```python
from build123d import *

# Parameters (mm, degrees)
F1_DEPTH = 4.75
F2_R     = 1.7
F3_DEPTH = 2.111
F4_R     = 1.6
F5_DEPTH = 2.111


with BuildPart() as f1:
    # F0 (on Front) → F1 (new body, symmetric)
    with BuildSketch(Plane.XZ):
        Polygon((-1.45, -4.75), (1.45, -4.75), (1.45, -3.15), (0.66, -3.15), (0.66, 0.05), (1.45, 0.05), (1.45, 1.65), (0.66, 1.65), (0.66, 4.75), (-1.45, 4.75), align=None)
    extrude(amount=F1_DEPTH, both=True)

    # F2 (on face) → F3 (cut, through all)
    with BuildSketch(Plane.YZ.offset(0.66)):
        with Locations((0, 4.75)):
            Circle(F2_R)
    extrude(amount=-F3_DEPTH, mode=Mode.SUBTRACT)

    # F4 (on face) → F5 (cut, through all)
    with BuildSketch(Plane.YZ.offset(0.66)):
        with Locations((0, -1.55)):
            Circle(F4_R)
    extrude(amount=-F5_DEPTH, mode=Mode.SUBTRACT)


solid = f1.part
```
Input: part model. Units: mm. Frame: model coordinates. A direction names the side the tool comes from. Coordinates: 2 decimals unless noted, no trailing zeros. Write each loop counter-clockwise with the first axis right and the second up, starting at its lowest first coordinate (ties: lowest second). Pieces come first, ordered by that corner, then holes. Notation, with made-up numbers: M 37,74.5 L 62,74.5 A21 cw 62,92.5 Z; hole C -22.75,23.25 d1. An arc over 180 degrees is marked long. Use one line per item in the form item = value.
Q1. First-contact query: pin 1 (0.9 mm diameter, centred on x = 1, y = 1, fed in from +Z); pin 2 (2.5 mm diameter, centred on y = -1.5, z = 3.5, fed in from +X). Flat tips, straight axial feed; report the tip coordinate or a pass-through.
Answer below:
pin_1 = 3.65
pin_2 = 0.66
Q2. Section A-A (z = -1.55). Return loops of the section in (x, y).
Answer below:
outline = M -1.45,-4.75 L 0.66,-4.75 L 0.66,-1.6 L -1.45,-1.6 Z; M -1.45,1.6 L 0.66,1.6 L 0.66,4.75 L -1.45,4.75 Z
Q3. Section B-B (x = 1). Return loops of the section in (y, z).
Answer below:
outline = M -4.75,-4.75 L 4.75,-4.75 L 4.75,-3.15 L -4.75,-3.15 Z; M -4.75,0.05 L 4.75,0.05 L 4.75,1.65 L -4.75,1.65 Z
Q4. Section D-D (z = 2.75). Return loops of the section in (x, y).
Answer below:
outline = M -1.45,-4.75 L 0.66,-4.75 L 0.66,4.75 L -1.45,4.75 Z
Q5. Material intervals for probe 1 along Z at (x, y) = (-0.6, 0); probe 2 along Y at (x, z) = (-0.8, -1.55); probe 3 along Z at (x, y) = (1.1, -3.75), sorted ascending. Write a range as from..to.
Answer below:
probe_1 = -4.75..-3.15, 0.05..3.05
probe_2 = -4.75..-1.6, 1.6..4.75
probe_3 = -4.75..-3.15, 0.05..1.65
Q6. Set-up query: faces 1 (the face through (0.66, -3, -2)), 2 (the face through (0, 4.75, 0)), 3 (the face through (0.66, -0.1, 2.8)). Return all of +Z, -Z, +X, -X, +Y, -Y with unobstructed straight access to the full face (end or side cutting, diameter ignored); none if empty.
Answer below:
face_1 = +X, +Y, -Y
face_2 = +Z, -Z, +X, -X, +Y
face_3 = +Z, +X, +Y, -Y
Q7. Section C-C (y = 2). Return loops of the section in (x, z).
Answer below:
outline = M -1.45,-4.75 L 1.45,-4.75 L 1.45,-3.15 L 0.66,-3.15 L 0.66,0.05 L 1.45,0.05 L 1.45,1.65 L 0.66,1.65 L 0.66,4.75 L -1.45,4.75 Z
